The listing builds one solid part. Answer for the finished solid, in the listing's coordinates (mm). A direction names the side the tool comes from. Coordinates: 2 decimals unless noted, no trailing zeros. Order: outer loops, then holes, each group sorted by start corner. A loop starts at its lowest first (then second) coordinate and runs counter-clockwise, first axis right, second up. Notation, with made-up numbers: (89, 53.5) - (113, 53.5) arc R8 cw to (113, 64.5) - close; hole circle Ø5 at (18.5, 59.5). An arc over 180 degrees is marked (long way). One line per item, written item: value. Start each with the question number.
```python
from build123d import *

# Parameters (mm, degrees)
SKETCH1_W               = 65
SKETCH1_H               = 90
SKETCH1_R               = 2.05
BOSS_EXTRUDE1_DEPTH     = 10
MIRROR2_COPY_1_SKETCH_W = 65
MIRROR2_COPY_1_SKETCH_H = 90
MIRROR2_COPY_1_SKETCH_R = 2.05
MIRROR2_COPY_1_DEPTH    = 10
SKETCH2_W               = 40.1
SKETCH2_H               = 5.1
CUT_EXTRUDE1_DEPTH      = 10
SKETCH3_R               = 1.55
CUT_EXTRUDE2_DEPTH      = 10


with BuildPart() as part:
    # Sketch1 → Boss-Extrude1 (new body)
    with BuildSketch(Plane(origin=(0, 0, 0), x_dir=(1, 0, 0), z_dir=(0, 1, 0))):
        with Locations((-32.5, 45)):
            Rectangle(SKETCH1_W, SKETCH1_H)
        with Locations((-50, 77)):
            Circle(SKETCH1_R, mode=Mode.SUBTRACT)
        with Locations((-50, 34.9)):
            Circle(SKETCH1_R, mode=Mode.SUBTRACT)
        with Locations((-50, 60)):
            Circle(SKETCH1_R, mode=Mode.SUBTRACT)
    boss_extrude1 = extrude(amount=BOSS_EXTRUDE1_DEPTH)

    # Mirror1: Boss-Extrude1 across Right Plane
    add(boss_extrude1.mirror(Plane(origin=(0, 0, 0), x_dir=(0, 0, -1), z_dir=(1, 0, 0))))

    # Mirror2: Boss-Extrude1 across Front Plane
    add(boss_extrude1.mirror(Plane.XY))

    # Mirror2 copy 1 sketch → Mirror2 copy 1 (add)
    with BuildSketch(Plane(origin=(0, 0, 0), x_dir=(-1, 0, 0), z_dir=(0, 1, 0))):
        with Locations((-32.5, 45)):
            Rectangle(MIRROR2_COPY_1_SKETCH_W, MIRROR2_COPY_1_SKETCH_H)
        with Locations((-50, 77)):
            Circle(MIRROR2_COPY_1_SKETCH_R, mode=Mode.SUBTRACT)
        with Locations((-50, 34.9)):
            Circle(MIRROR2_COPY_1_SKETCH_R, mode=Mode.SUBTRACT)
        with Locations((-50, 60)):
            Circle(MIRROR2_COPY_1_SKETCH_R, mode=Mode.SUBTRACT)
    extrude(amount=MIRROR2_COPY_1_DEPTH)

    # Sketch2 → Cut-Extrude1 (cut)
    with BuildSketch(Plane(origin=(0, 10, 0), x_dir=(1, 0, 0), z_dir=(0, 1, 0))):
        with Locations((0, 7.55)):
            Rectangle(SKETCH2_W, SKETCH2_H)
        with Locations((0, -7.55)):
            Rectangle(SKETCH2_W, SKETCH2_H)
    extrude(amount=-CUT_EXTRUDE1_DEPTH, mode=Mode.SUBTRACT)

    # Sketch3 → Cut-Extrude2 (cut)
    with BuildSketch(Plane(origin=(0, 10, 0), x_dir=(1, 0, 0), z_dir=(0, 1, 0))):
        with Locations((-23.55, 86.6)):
            Circle(SKETCH3_R)
        with Locations((-23.55, 23.55)):
            Circle(SKETCH3_R)
        with Locations((-61.5, 23.55)):
            Circle(SKETCH3_R)
        with Locations((23.55, 23.55)):
            Circle(SKETCH3_R)
        with Locations((23.55, 86.6)):
            Circle(SKETCH3_R)
        with Locations((61.5, 23.55)):
            Circle(SKETCH3_R)
        with Locations((-61.5, -23.55)):
            Circle(SKETCH3_R)
        with Locations((0, -23.55)):
            Circle(SKETCH3_R)
        with Locations((61.5, -23.55)):
            Circle(SKETCH3_R)
    extrude(amount=-CUT_EXTRUDE2_DEPTH, mode=Mode.SUBTRACT)


solid = part.part
```
(1) For faces 1 (the face through (1, 10, 1)), 2 (the face through (20.05, 5, 8)), determine the directions among +Z, -Z, +X, -X, +Y, -Y from which every point of the face is accessible in a straight line to the end or side of a thin tool.
(2) The part is cut by section A-A on z = 77. Determine the outline of the cut face in (x, y), plus the area to 3 significant figures.
(3) The part is cut by section D-D on y = 1.5. Count the separate pieces of the cut face and the enclosed holes in it, plus the area to 3 significant figures.
(4) The part is cut by section C-C on x = -50. Determine the outline of the cut face in (y, z).
(5) Flat-ended cylindrical pins translate along their axes: pin 1 Ø3.5 at (x, z) = (-50, -60) entering from -Y; pin 2 Ø5 at (x, z) = (23.55, -23.55) entering from +Y. Find the tip coordinate at first contact, or state that the pin passes through.
(6) Consider probe 1 along X at (y, z) = (3, -77); probe 2 along Z at (x, y) = (6, 1.5); probe 3 along Z at (x, y) = (23.55, 4.25). Determine where each line is inside the solid, lowest interval first.
(7) The part is cut by section B-B on x = -17. Determine the outline of the cut face in (y, z), plus the area to 3 significant figures.
(8) For a pull along X with two mould halves and no side action, classify faces 3 (the face through (-65, 5, -1)), 4 (the face through (1, 5, 90)), 5 (the face through (-51.5, 4.9, -61.4)) as pulls with the +X half, pulls with the -X half, needs draft (parallel to the pull), parting line crosses it, or undercut.
Completed:
1. face 1: +Z, -Z, +X, -X, +Y
1. face 2: +Y, -Y
2. outline: (-65, 0) - (-52.05, 0) - (-52.05, 10) - (-65, 10) - close; (-47.95, 0) - (47.95, 0) - (47.95, 10) - (-47.95, 10) - close; (52.05, 0) - (65, 0) - (65, 10) - (52.05, 10) - close
2. area: 1,220 mm2
3. separate pieces: 1
3. enclosed holes: 23
3. area: 22,800 mm2
4. outline: (0, -90) - (10, -90) - (10, -79.05) - (0, -79.05) - close; (0, -74.95) - (10, -74.95) - (10, -62.05) - (0, -62.05) - close; (0, -57.95) - (10, -57.95) - (10, -36.95) - (0, -36.95) - close; (0, -32.85) - (10, -32.85) - (10, 32.85) - (0, 32.85) - close; (0, 36.95) - (10, 36.95) - (10, 57.95) - (0, 57.95) - close; (0, 62.05) - (10, 62.05) - (10, 74.95) - (0, 74.95) - close; (0, 79.05) - (10, 79.05) - (10, 90) - (0, 90) - close
5. pin 1: passes through
5. pin 2: stops at y = 10
6. probe 1: x = -65 to -52.05, -47.95 to 47.95, 52.05 to 65
6. probe 2: z = -90 to -10.1, -5 to 5, 10.1 to 90
6. probe 3: z = -90 to -88.15, -85.05 to -25.1, -22 to 90
7. outline: (0, -90) - (10, -90) - (10, -10.1) - (0, -10.1) - close; (0, -5) - (10, -5) - (10, 5) - (0, 5) - close; (0, 10.1) - (10, 10.1) - (10, 90) - (0, 90) - close
7. area: 1,700 mm2
8. face 3: pulls with the -X half
8. face 4: needs draft
8. face 5: undercut
